from build123d import *

# Parameters (mm, degrees)
SKETCH_W        = 38
SKETCH_H        = 80
PAD_DEPTH       = 20
SKETCH001_W     = 5
SKETCH001_H     = 5
POCKET_DEPTH    = 5
SKETCH002_W     = 5.01717
SKETCH002_H     = 4.6615971845
POCKET001_DEPTH = 2
FILLET_R        = 1


with BuildPart() as part:
    # Sketch → Pad (new body)
    with BuildSketch(Plane.XY):
        with Locations((19, 40)):
            Rectangle(SKETCH_W, SKETCH_H)
    extrude(amount=PAD_DEPTH)

    # Sketch001 (on Face6 of Pad) → Pocket (cut)
    with BuildSketch(Plane.XY.offset(20)):
        with Locations((35.5, 72.8384028155)):
            Rectangle(SKETCH001_W, SKETCH001_H)
    extrude(amount=-POCKET_DEPTH, mode=Mode.SUBTRACT)

    # Sketch002 (on Face5 of Pocket) → Pocket001 (cut)
    with BuildSketch(Plane.XY.offset(20)):
        with Locations((35.491415, 77.6692014078)):
            Rectangle(SKETCH002_W, SKETCH002_H)
    extrude(amount=-POCKET001_DEPTH, mode=Mode.SUBTRACT)

    # Fillet
    fillet_edges = [part.edges().sort_by_distance(p)[0] for p in [
        (35.491415, 80, 18),
    ]]
    fillet(fillet_edges, radius=FILLET_R)


solid = part.part
Here's how the part is built. I have some questions about the finished solid (model axes, mm). A direction names the side the tool comes from. Round coordinates to 2 decimals unless told otherwise and drop trailing zeros. Order: outer loops, then holes, each group sorted by start corner. A loop starts at its lowest first (then second) coordinate and runs counter-clockwise, first axis right, second up. Notation, with made-up numbers: (43.25, -30) -> (85.25, -30) arc R16 ccw to (85.25, -4) -> close; hole circle Ø4 at (60.5, 60). An arc over 180 degrees is marked (long way). Use CSV: the item, a comma, the result in double quotes.
1. I'm going to push flat-ended pins straight in: P1, Ø2.5, axis at y = 72, z = 16.5, coming from the +X side; P2, Ø2.5, axis at x = 36, y = 72.5, coming from the +Z side. Where does each tip first touch, or does it pass through?
Recorded:
P1,"stops at x = 33"
P2,"stops at z = 15"
2. I want a section at A-A on x = 34.5. List the corners of the cut face in (y, z) for me.
Recorded:
outline,"(0, 0) -> (80, 0) -> (80, 17) arc R1 ccw to (79, 18) -> (75.34, 18) -> (75.34, 15) -> (70.34, 15) -> (70.34, 20) -> (0, 20) -> close"
3. Which directions (+Z, -Z, +X, -X, +Y, -Y) give clear straight access to the entire face, cutting with the end or side of a thin tool? Please do faces 5 (the face through (32.983, 78, 19)), 6 (the face through (38, 39, 10)), 7 (the face through (35, 75.338, 17)).
Recorded:
face 5,"+Z, +X, +Y"
face 6,"+Z, -Z, +X, +Y, -Y"
face 7,"+Z, +X"
4. Thinking about a two-plate mould opening in Y: for faces 1 (the face through (35, 70.338, 18)), 2 (the face through (19, 80, 10)), 3 (the face through (19, 41, 20)), 4 (the face through (33, 73, 18)), which applies, pulls with the +Y half, pulls with the -Y half, needs draft (parallel to the pull), parting line crosses it, or undercut?
Recorded:
face 1,"undercut"
face 2,"pulls with the +Y half"
face 3,"needs draft"
face 4,"undercut"
